Autodesk Inventor part; units mm, degrees
ref_plane "YZ Plane" through (0, 0, 0) normal (1, 0, 0) x (0, 1, 0)
ref_plane "XZ Plane" through (0, 0, 0) normal (0, 1, 0) x (-1, 0, 0)
ref_plane "XY Plane" through (0, 0, 0) normal (0, 0, 1) x (1, 0, 0)
sketch "Sketch1" plane through (0, 0, 0) normal (0, 1, 0) x (-1, 0, 0)
  circle A0 centre (-7.5, 4.5) radius 1
  circle A1 centre (-7.5, 9.5) radius 1
  circle A2 centre (-7.5, 18.84) radius 0.6
  circle A3 centre (-7.5, 29.5) radius 2.5
  circle A4 centre (-7.5, 29.576) radius 6.0215
  circle A5 centre (-7.5, 29.576) radius 4.0045
  circle A6 centre (-7.5, 3.274) radius 3.274
  circle A7 centre (-7.5, 15.5) radius 2.5045
  line L0 (-7.5, 3.274) -> (-7.5, 29.576)
  line L1 (-3.5183, 29.1493) -> (-5.0098, 15.2331)
  line L2 (-9.9902, 15.2331) -> (-11.4817, 29.1493)
  line L3 (-1.5114, 28.947) -> (-4.2439, 2.932)
  line L4 (-13.4886, 28.947) -> (-10.7561, 2.932)
  line L5 (-1.5114, 28.947) -> (-3.5183, 29.1493)
  line L6 (-13.4886, 28.947) -> (-11.4817, 29.1493)
  line L7 (-3.4324, 10.6581) -> (-11.5347, 10.3447)
  line L8 (-3.3796, 11.1605) -> (-11.587, 10.843)
  point P0 (0, 0)
  point P1 (-7.5, 10.5007)
  point P2 (-7.5, 10.5)
  point P3 (-7.5387, 10.4993)
  dimension "d2" = 2
  dimension "d3" = 2
  dimension "d4" = 1.2
  dimension "d5" = 5
  dimension "d6" = 12.043
  dimension "d7" = 8.009
  dimension "d8" = 6.548
  dimension "d9" = 5.009
  dimension "d10" = 5
  dimension "d11" = 1.226
  dimension "d12" = 6
  dimension "d15" = 26.302
  dimension "d16" = 3.34
  dimension "d17" = 10.66
  dimension "d18" = 26.302
  dimension "d19" = 25
  dimension "d28" = 0.5
extrude "Extrusion1" add sketch "Sketch1" along normal blind 4.7 contours A4 L5 A5 L6
extrude "Extrusion2" add sketch "Sketch1" along normal blind 2.7 contours A6 | A6 L4 L7 A1 L0 | L0 A1 L7 L3 A6 | L4 L8 L0 L7 | L0 L8 L3 L7 | L4 A4 L2 A7 L0 L8 | L0 A7 L1 A4 L3 L8 | L6 L2 A4 | A4 L1 L5
extrude "Extrusion3" add sketch "Sketch1" along normal blind 1.2 contours L0 A7 | A7 L0 | L2 A5 L0 A4 | A4 L0 A2 A7 L2 | A5 | A7 L0 A2 A4 L1 | A4 L0 A5 L1
extrude "Extrusion4" add sketch "Sketch1" along normal blind 7.1 contours A6 | A6 L4 L7 A1 L0 | L0 A1 L7 L3 A6 | L4 L8 L0 L7 | L0 L8 L3 L7
properties part number "servoarm"
CAD build for the part. Positions are in the model's coordinates, mm. A direction names the side the tool comes from. Give positions to 0.01 mm unless a question says otherwise; leave off trailing zeros. Order: outer loops, then holes, each group sorted by start corner. A loop starts at its lowest first (then second) coordinate and runs counter-clockwise, first axis right, second up.
(1) Saw through at D-D, the plane y = 0.5. Give the cut face in (x, z), then the cut area to 3 significant figures.
(2) Tool access for faces 4 (the cylindrical face through (7.22, 0.59, 19.37)), 5 (the cylindrical face through (7.59, 2.93, 33.58)): list every direction of +Z, -Z, +X, -X, +Y, -Y with a clear straight run to the whole face (end or side of a thin tool).
(3) Saw through at A-A, the plane y = 4. Give the cut face in (x, z).
(4) Saw through at B-B, the plane z = 18.84. Give the cut face in (x, y).
(5) Mould opens along X. For faces 1 (the cylindrical face through (7.641, 2.317, 35.596)), 2 (the flat face through (8, 4.7, 34)), 3 (the flat face through (2.501, 3.686, 29.047)) say: released by +X, released by -X, zero draft, split by the parting line, or undercut.
(6) Drill centre lines: L1, parallel to Z at x = 7.5, y = 2; L2, parallel to Z at x = 7.5, y = 3.45; L3, parallel to Z at x = 7.5, y = 0.85. Where is each one in solid material? Low to high.
(7) Saw through at C-C, the plane y = 5.5. Give the cut face in (x, z).
(8) Flat gauge pins, fed straight in: pin 1 (4 mm diameter, centred on x = 6, z = 19, fed in from +Y); pin 2 (5.5 mm diameter, centred on x = 6, z = 32.5, fed in from +Y); pin 3 (4 mm diameter, centred on y = 6, z = 18.5, fed in from +X); pin 4 (7 mm diameter, centred on x = 7.5, z = 29.576, fed in from +Y). Where does each tip first touch, or does it go through?
Results found:
1. outline: (1.51, 28.95) - (4.24, 2.93) arc R3.27 ccw to (10.76, 2.93) - (13.49, 28.95) arc R6.02 ccw (long way) to start; hole circle Ø5 at (7.5, 29.5); hole circle Ø2 at (7.5, 4.5); hole circle Ø2 at (7.5, 9.5); hole circle Ø1.2 at (7.5, 18.84)
1. area: 293 mm2
2. face 4: +Y, -Y
2. face 5: +Y
3. outline: (1.51, 28.95) - (3.52, 29.15) arc R4 cw (long way) to (11.48, 29.15) - (13.49, 28.95) arc R6.02 ccw (long way) to start; (3.38, 11.16) - (4.24, 2.93) arc R3.27 ccw to (10.76, 2.93) - (11.59, 10.84) - close; hole circle Ø2 at (7.5, 4.5); hole circle Ø2 at (7.5, 9.5)
4. outline: (2.57, 0) - (6.9, 0) - (6.9, 1.2) - (4.62, 1.2) - (4.62, 2.7) - (2.57, 2.7) - close; (8.1, 0) - (12.43, 0) - (12.43, 2.7) - (10.38, 2.7) - (10.38, 1.2) - (8.1, 1.2) - close
5. face 1: split by the parting line
5. face 2: zero draft
5. face 3: undercut
6. L1: z = 0 to 3.5, 5.5 to 8.5, 10.5 to 13, 33.58 to 35.6
6. L2: z = 0 to 3.5, 5.5 to 8.5, 10.5 to 11, 33.58 to 35.6
6. L3: z = 0 to 3.5, 5.5 to 8.5, 10.5 to 18.24, 19.44 to 27, 32 to 35.6
7. outline: (3.38, 11.16) - (4.24, 2.93) arc R3.27 ccw to (10.76, 2.93) - (11.59, 10.84) - close; hole circle Ø2 at (7.5, 4.5); hole circle Ø2 at (7.5, 9.5)
8. pin 1: stops at y = 2.7
8. pin 2: stops at y = 4.7
8. pin 3: passes through
8. pin 4: stops at y = 1.2
